Source: CAD feature listing. Evaluate the final solid. Frame: model axes, mm. Face numbers are marked on the shaded views. A direction names the side the tool comes from. Coordinates: 2 decimals unless noted, no trailing zeros. Loops run counter-clockwise (first coordinate to the right, second up) from the corner with the lowest first, then second, coordinate; pieces in that order, holes last. Notation, with made-up numbers: M -20,-21.5 L 20,-21.5 A32 cw 20,15.5 Z; hole C 13.5,76 d9. An arc over 180 degrees is marked long. One line per question, with ' | ' between items. Start each with the question number.
1. Section query B-B, the plane x = 0. Output: boundary loops of the cut face in (y, z), and give its area (3 significant figures).
2. Access query for the marked faces 1, 2 and 3. Directions: +Z, -Z, +X, -X, +Y, -Y. A direction counts if a zero-diameter tool reaches every point of the face in a straight line with its end or side. Return the directions, or none.
3. Ray query, probe 1 along Y at (x, z) = (1.5, 4.5); probe 2 along Y at (x, z) = (11, 4.75); probe 3 along Z at (x, y) = (4.5, -5). Return the intervals inside material, ascending.
4. Section query A-A, the plane x = 9.5. Output: boundary loops of the cut face in (y, z).
5. Pin query (flat end, axial travel): P1, Ø4, axis at x = -1.5, y = 6.5, coming from the +Z side; P2, Ø6, axis at x = 3.5, y = -6, coming from the +Z side; P3, Ø10, axis at x = -8.5, y = -2, coming from the +Z side. Return the tip coordinate at first contact, or that it passes through.
```python
from build123d import *

# Parameters (mm, degrees)
FILLET1_R     = 2.54
CHAMFER1_SIZE = 0.508


with BuildPart() as part:
    # Sketch1 → Revolve1 (revolve)
    with BuildSketch(Plane.XY, mode=Mode.PRIVATE) as revolve1_sk:
        with BuildLine():
            Line((-12.6746, 6.35), (12.6746, 6.35))
            Line((12.6746, 6.35), (12.6746, 7.62))
            Line((12.6746, 7.62), (6.329647384, 7.62))
            ThreePointArc((6.329647384, 7.62), (0, 9.906), (-6.329647384, 7.62))
            Line((-6.329647384, 7.62), (-12.6746, 7.62))
            Line((-12.6746, 7.62), (-12.6746, 6.35))
        make_face()
    revolve(revolve1_sk.sketch.rotate(Axis((-29.740184884, 0, 0), (1, 0, 0)), 90), axis=Axis((-29.740184884, 0, 0), (1, 0, 0)))

    # Fillet1
    fillet1_edges = [part.edges().sort_by_distance(p)[0] for p in [
        (-6.329647384, 0, -7.62),
        (6.329647384, 0, -7.62),
    ]]
    fillet(fillet1_edges, radius=FILLET1_R)

    # Chamfer1
    chamfer1_edges = [part.edges().sort_by_distance(p)[0] for p in [
        (12.6746, 0, -6.35),
        (-12.6746, 0, -6.35),
    ]]
    chamfer(chamfer1_edges, length=CHAMFER1_SIZE)


solid = part.part
```
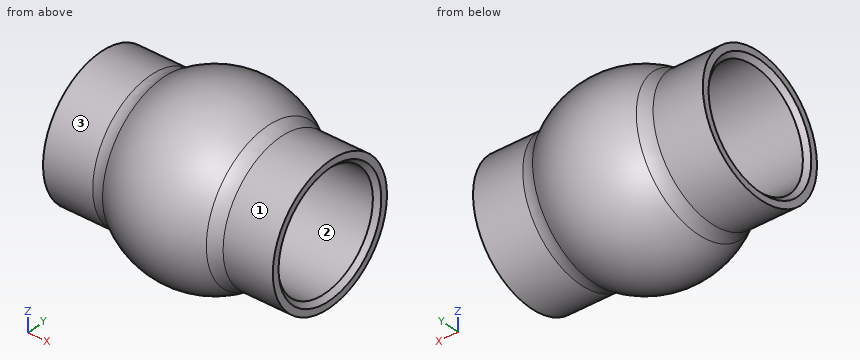
Taken from the geometry:
1) outline: C 0,0 d19.81; hole C 0,0 d12.7 | area: 182 mm^2
2) face 1: +X | face 2: +X, -X | face 3: -X
3) probe 1: -8.7 to -4.48, 4.48 to 8.7 | probe 2: -5.96 to -4.21, 4.21 to 5.96 | probe 3: -7.27 to -3.91, 3.91 to 7.27
4) outline: C 0,0 d15.24; hole C 0,0 d12.7
5) P1: z = 8.74 | P2: z = 9.09 | P3: z = 9.18
